```python
from build123d import *

# Parameters (mm, degrees)
SKETCH1_W           = 30
SKETCH1_H           = 38
BOSS_EXTRUDE1_DEPTH = 3.175
SKETCH2_W           = 30
SKETCH2_H           = 3.175
BOSS_EXTRUDE2_DEPTH = 34.825
SKETCH3_R           = 4
CUT_EXTRUDE1_DEPTH  = 60.638751035
SKETCH4_R           = 4
CUT_EXTRUDE2_DEPTH  = 58.667679423


with BuildPart() as part:
    # Sketch1 → Boss-Extrude1 (new body)
    with BuildSketch(Plane.XY):
        with Locations((15, 19)):
            Rectangle(SKETCH1_W, SKETCH1_H)
    extrude(amount=BOSS_EXTRUDE1_DEPTH)

    # Sketch2 → Boss-Extrude2 (add)
    with BuildSketch(Plane(origin=(0, 0, 0), x_dir=(-1, 0, 0), z_dir=(0, 0, -1))):
        with Locations((-15, 1.5875)):
            Rectangle(SKETCH2_W, SKETCH2_H)
    extrude(amount=BOSS_EXTRUDE2_DEPTH)

    # Sketch3 → Cut-Extrude1 (cut, through all)
    with BuildSketch(Plane(origin=(0, 0, 0), x_dir=(-1, 0, 0), z_dir=(0, 0, -1))):
        with Locations((-15, 27)):
            Circle(SKETCH3_R)
    extrude(amount=-CUT_EXTRUDE1_DEPTH, mode=Mode.SUBTRACT)

    # Sketch4 → Cut-Extrude2 (cut, through all)
    with BuildSketch(Plane(origin=(0, 3.175, 0), x_dir=(1, 0, 0), z_dir=(0, 1, 0))):
        with Locations(Location((15, 11.825, 0), (0, 0, 180))):
            Circle(SKETCH4_R)
    extrude(amount=-CUT_EXTRUDE2_DEPTH, mode=Mode.SUBTRACT)


solid = part.part
```
Geometry: final body of the model. Coordinates: model frame, mm. A direction names the side the tool comes from. Round coordinates to 2 decimals unless told otherwise and drop trailing zeros. Order: outer loops, then holes, each group sorted by start corner. A loop starts at its lowest first (then second) coordinate and runs counter-clockwise, first axis right, second up. Notation, with made-up numbers: (82, -22) -> (117, -22) arc R9 ccw to (117, -15) -> close; hole circle Ø4 at (32.25, 68.5). An arc over 180 degrees is marked (long way). Use one line per item in the form item = value.
(1) Section D-D on y = 14. Return loops of the section in (x, z) (3 decimals), and give its area (4 significant figures).
Results list:
outline = (0, 0) -> (30, 0) -> (30, 3.175) -> (0, 3.175) -> close
area = 95.25 mm^2
(2) Section C-C on x = 2. Return loops of the section in (y, z) (3 decimals).
Results list:
outline = (0, -34.825) -> (3.175, -34.825) -> (3.175, 0) -> (38, 0) -> (38, 3.175) -> (0, 3.175) -> close
(3) Ray query, probe 1 along Z at (x, y) = (8.75, 27) (3 decimals). Return the intervals inside material, ascending. Write a range as [from, to].
Results list:
probe_1 = [0, 3.175]
(4) Draft query along X for faces 1 (the face through (30, 2, -7)), 2 (the face through (17.95, 29.7, 1.57)), 3 (the face through (15, 2, -34.825)). Return one class per face: pulls with the +X half, pulls with the -X half, needs draft (parallel to the pull), parting line crosses it, or undercut.
Results list:
face_1 = pulls with the +X half
face_2 = undercut
face_3 = needs draft
(5) Section B-B on y = 27. Return loops of the section in (x, z) (3 decimals).
Results list:
outline = (0, 0) -> (11, 0) -> (11, 3.175) -> (0, 3.175) -> close; (19, 0) -> (30, 0) -> (30, 3.175) -> (19, 3.175) -> close
(6) First-contact query: pin 1 Ø9 at (x, y) = (9.5, 28) entering from -Z; pin 2 Ø3 at (x, z) = (11.5, -18) entering from +Y (3 decimals). Flat tips, straight axial feed; report the tip coordinate or a pass-through.
Results list:
pin_1 = 0
pin_2 = 3.175
(7) Section A-A on x = 15. Return loops of the section in (y, z) (3 decimals), and give its area (3 significant figures).
Results list:
outline = (0, -34.825) -> (3.175, -34.825) -> (3.175, -15.825) -> (0, -15.825) -> close; (0, -7.825) -> (3.175, -7.825) -> (3.175, 0) -> (23, 0) -> (23, 3.175) -> (0, 3.175) -> close; (31, 0) -> (38, 0) -> (38, 3.175) -> (31, 3.175) -> close
area = 180 mm^2
(8) Access query for faces 4 (the face through (15, 3.175, -17)), 5 (the face through (15, 19, 3.175)). Directions: +Z, -Z, +X, -X, +Y, -Y. A direction counts if a zero-diameter tool reaches every point of the face in a straight line with its end or side. Return the directions, or none.
Results list:
face_4 = -Z, +X, -X, +Y
face_5 = +Z, +X, -X, +Y, -Y
